Input: part model. Units: mm. Frame: model coordinates. Face numbers are marked on the shaded views. A direction names the side the tool comes from. Give positions to 0.01 mm unless a question says otherwise; leave off trailing zeros. Write each loop counter-clockwise with the first axis right and the second up, starting at its lowest first coordinate (ties: lowest second). Pieces come first, ordered by that corner, then holes. Notation, with made-up numbers: M 44.25,38.25 L 87.25,38.25 A36 ccw 87.25,75.25 Z; hole C 85,-31.5 d7. An arc over 180 degrees is marked long. Use CSV: the item, a comma, the result in double quotes. Start each with the question number.
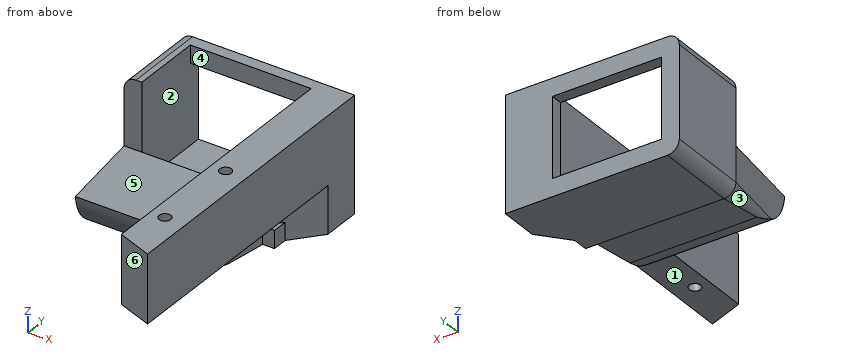
Autodesk Inventor part; units mm, degrees
ref_plane "作業平面1" through (0, 45, -9.5) normal (1, 0, 0) x (0, 0, -1)
ref_plane "作業平面2" through (3, 2, -11.5) normal (0, 0, -1) x (-1, 0, 0)
ref_plane "YZ Plane" through (0, 0, 0) normal (1, 0, 0) x (0, 1, 0)
sketch "スケッチ1" plane through (0, 0, 0) normal (1, 0, 0) x (0, 1, 0)
  line L0 (45, 0) -> (0, 0)
  line L1 (0, 0) -> (0, -11.5)
  line L2 (0, -11.5) -> (45, -11.5)
  line L3 (45, -11.5) -> (45, 0)
  dimension "d0" = 45
  dimension "d1" = 11.5
extrude "押し出し1" add sketch "スケッチ1" along normal blind 3
sketch "スケッチ5" plane through (0, 45, 0) normal (0, 1, 0) x (1, 0, 0)
  line L0 (-5, 3) -> (-23.5, 3)
  line L1 (-23.5, 3) -> (-23.5, 16.5)
  line L2 (-23.5, 16.5) -> (-5, 16.5)
  line L3 (-5, 16.5) -> (-5, 3)
  line L4 (0, 0) -> (-26.5, 0)
  line L5 (-26.5, 0) -> (-26.5, 19.5)
  line L6 (-26.5, 19.5) -> (0, 19.5)
  line L7 (0, 19.5) -> (0, 0)
  point P0 (3, 0)
  dimension "d15" = 18.5
  dimension "d16" = 13.5
  dimension "d17" = 3
  dimension "d18" = 5
  dimension "d19" = 3
  dimension "d20" = 3
extrude "押し出し4" add sketch "スケッチ5" against normal blind 2
ref_plane "作業平面1" through (0, 45, -9.5) normal (1, 0, 0) x (0, 0, -1)
sketch "スケッチ7" plane through (0, 45, -9.5) normal (1, 0, 0) x (0, 0, -1)
  line L0 (0, 0) -> (10, 0)
  line L1 (10, -2) -> (2, -2)
  line L2 (10, 0) -> (10, -2)
  line L3 (2, 0) -> (10, 0)
  line L4 (2, -2) -> (2, 0)
  point P0 (-9.5, -45)
extrude "押し出し6" cut sketch "スケッチ7" against normal blind 1
fillet "フィレット2" radius 2 2 edges at (-26.5, 44, 0) (-26.5, 44, -19.5)
sketch "スケッチ8" plane through (0, 0, 0) normal (-1, 0, 0) x (0, 0, 1)
  line L0 (0, 43) -> (-11.5, 43)
  line L1 (-11.5, 0) -> (-11.5, 43)
  line L2 (0, 0) -> (-11.5, 0)
  line L3 (0, 43) -> (0, 0)
  line L4 (-3, 39.3409) -> (0, 39.3409)
  line L5 (0, 39.3409) -> (0, 27.7002)
  line L6 (0, 27.7002) -> (-3, 27.7002)
  line L7 (-3, 27.7002) -> (-3, 39.3409)
extrude "押し出し7" add sketch "スケッチ8" along normal blind 3
ref_plane "作業平面2" through (3, 2, -11.5) normal (0, 0, -1) x (-1, 0, 0)
sketch "スケッチ10" plane through (3, 2, -11.5) normal (0, 0, -1) x (-1, 0, 0)
  line L0 (-2, -9) -> (6, -6)
  line L1 (6, -6) -> (6, 22)
  line L2 (0, -2) -> (0, 0)
  line L3 (0, -2) -> (6, -2)
  line L4 (0, -2) -> (0, -8.25)
  point P0 (3, -2)
extrude "押し出し9" add sketch "スケッチ10" against normal up to surface (11.5 mm away)
sketch "スケッチ11" plane through (3, 45, -11.5) normal (0, 0, -1) x (-1, 0, 0)
  circle A0 centre (3.5, -26.8338) radius 1
  circle A1 centre (3.5, -41.8338) radius 1
  point P0 (3, -45)
sketch "スケッチ12" plane through (0, 43, 0) normal (0, -1, 0) x (1, 0, 0)
  line L0 (-1, -11.5) -> (-3, -11.5)
  line L1 (-3, -11.5) -> (-3, 0)
  line L2 (-3, 0) -> (-24.5, 0)
  arc A0 (-24.5, 0) -> (-26.5, -2) centre (-24.5, -2) ccw
  line L3 (-26.5, -2) -> (-26.5, -17.5)
  arc A1 (-26.5, -17.5) -> (-24.5, -19.5) centre (-24.5, -17.5) ccw
  line L4 (-24.5, -19.5) -> (-1, -19.5)
  line L5 (-1, -19.5) -> (-1, -11.5)
  line L6 (-23.5, -3) -> (-5, -3)
  line L7 (-5, -3) -> (-5, -16.5)
  line L8 (-5, -16.5) -> (-23.5, -16.5)
  line L9 (-23.5, -16.5) -> (-23.5, -3)
  line L10 (-5, -16.5) -> (-1, -16.5)
  line L11 (-23.5, -3) -> (-23.5, 0)
  line L12 (-3, -11.5) -> (-5, -16.5)
  point P0 (0, 0)
extrude "押し出し10" add sketch "スケッチ12" along normal blind 12 contours L5 L4 A1 L3 A0 L2 L11 L9 L8 L10
sketch "スケッチ13" plane through (3, 45, -11.5) normal (0, 0, -1) x (-1, 0, 0)
  line L0 (6, -16.8338) -> (-2.2366, -7.0996)
  line L1 (6, -2) -> (6, -49)
  line L2 (4, -2) -> (6, -2)
  line L3 (4, -2) -> (4, 0)
  line L4 (4, 0) -> (0, 0)
  line L5 (0, 0) -> (0, -51.25)
  line L6 (0, -51.25) -> (6, -49)
  line L7 (0, -6.6466) -> (6, -13.7375)
  line L8 (6, -49) -> (6, -2)
  point P0 (3, -45)
  point P1 (6, -13.7375)
  dimension "d38" = 2
extrude "押し出し11" add sketch "スケッチ13" along normal up to surface (8 mm away) contours L7 L5 L4 L3 L2 L1
sketch "スケッチ14" plane through (0, 31, 0) normal (0, -1, 0) x (1, 0, 0)
  line L0 (-1, -19.5) -> (-1, -16.5)
  line L1 (-1, -16.5) -> (-23.5, -16.5)
  line L2 (-23.5, -16.5) -> (-23.5, 0)
  line L3 (-23.5, 0) -> (-24.5, 0)
  arc A0 (-24.5, 0) -> (-26.5, -2) centre (-24.5, -2) ccw
  line L4 (-26.5, -2) -> (-26.5, -17.5)
  arc A1 (-26.5, -17.5) -> (-24.5, -19.5) centre (-24.5, -17.5) ccw
  line L5 (-24.5, -19.5) -> (-1, -19.5)
  line L6 (-1, -19.5) -> (-26.5, -19.5)
  line L7 (-26.5, -19.5) -> (-26.5, -11.5)
  line L8 (-26.5, -11.5) -> (-1, -11.5)
  line L9 (-1, -11.5) -> (-1, -19.5)
  line L10 (-3, -11.5) -> (-3, -16.5)
  line L11 (-3, -16.5) -> (-3, -19.5)
  point P0 (0, 0)
  dimension "d41" = 8
extrude "押し出し12" add sketch "スケッチ14" along normal blind 15 contours L5 A1 L4 L8 L2 L1 L11 | L1 L2 L8 L10
chamfer "面取り1" distance 2 distance2 15 3 edges at (-13.75, 16, -19.5) (-25.9142, 16, -18.9142) (-26.5, 16, -14.5) measured on face at (-18, 16, -14.1667)
fillet "フィレット3" radius 8 1 edges at (-13.75, 16, -17.5001)
extrude "押し出し13" cut sketch "スケッチ11" against normal through all
equation "\"d19\" = d17"
equation "\"d20\" = d17"
properties part number "switch_setter"
Q1. Pull-direction query (X, two-part tool) for the marked faces 1, 2 and 3; classes: released by +X, released by -X, zero draft, split by the parting line, or undercut.
Q2. Section D-D, the plane y = 42. Return the cut outline in (x, z).
Q3. First-contact query: pin 1 Ø2 at (x, y) = (-8.5, 33.5) entering from +Z; pin 2 Ø2.5 at (x, y) = (-0.5, 3.17) entering from -Z; pin 3 Ø8 at (x, z) = (-7, -14) entering from -Y. Flat tips, straight axial feed; report the tip coordinate or a pass-through.
Q4. Section B-B, the plane z = -8.25. Return the cut outline in (x, y).
Q5. Section A-A, the plane x = -21.5. Return the cut outline in (y, z).
Q6. Material intervals for L1, parallel to Y at x = -0.5, z = -8.5; L2, parallel to Y at x = -1, z = -5.25; L3, parallel to X at y = -3, z = -2.25, sorted ascending. Write a range as [from, to].
Q7. Set-up query: the marked faces 4, 5 and 6. Return all of +Z, -Z, +X, -X, +Y, -Y with unobstructed straight access to the full face (end or side cutting, diameter ignored); none if empty.
Check result:
1,face 1,"zero draft"
1,face 2,"undercut"
1,face 3,"released by -X"
2,outline,"M -26.5,-17.5 A2 ccw -24.5,-19.5 L 3,-19.5 L 3,0 L -3,0 L -3,-16.5 L -23.5,-16.5 L -23.5,0 L -24.5,0 A2 ccw -26.5,-2 Z"
3,pin 1,"stops at z = -16.5"
3,pin 2,"stops at z = -11.5"
3,pin 3,"stops at y = 16"
4,outline,"M -26.5,31 L -23.5,31 L -23.5,45 L -26.5,45 Z; M -5,43 L -3,43 L -3,-4 L 3,-6.25 L 3,45 L -5,45 Z; hole C -0.5,3.17 d2; hole C -0.5,18.17 d2"
5,outline,"M 16,-11.5 A8 ccw 22.88,-18.42 L 31,-19.5 L 45,-19.5 L 45,-16.5 L 31,-16.5 L 31,-11.5 Z; M 43,-3 L 45,-3 L 45,0 L 43,0 Z"
6,L1,"y = [-4.94, 2.17], [4.17, 17.17], [19.17, 45]"
6,L2,"y = [-4.75, 2.3], [4.03, 17.3], [19.03, 45]"
6,L3,"x = [-3, 3]"
7,face 4,"+Z"
7,face 5,"+Z, -X, -Y"
7,face 6,"+Z, -Z, -X, -Y"
